Source: CAD feature listing. Evaluate the final solid. Frame: model axes, mm. A direction names the side the tool comes from. Round coordinates to 2 decimals unless told otherwise and drop trailing zeros. Order: outer loops, then holes, each group sorted by start corner. A loop starts at its lowest first (then second) coordinate and runs counter-clockwise, first axis right, second up. Notation, with made-up numbers: M 71,-4 L 109,-4 A11 ccw 109,11 Z; hole C 1,-16.5 d4. An arc over 180 degrees is marked long. Answer as CSV lines item,"result". Start each with the question number.
Item 1: First-contact query: P1, Ø3.5, axis at x = 0, y = 0, coming from the +Z side; P2, Ø2.5, axis at x = 0, y = 0, coming from the -Z side; P3, Ø2, axis at y = -2, z = 32, coming from the -X side; P4, Ø2, axis at x = 2, z = 22.5, coming from the -Y side. Flat tips, straight axial feed; report the tip coordinate or a pass-through.
Item 2: Set-up query: faces 1 (the face through (0, 0, 29)), 2 (the face through (0, 0, 6)), 3 (the face through (1.2, -1.2, 0)). Return all of +Z, -Z, +X, -X, +Y, -Y with unobstructed straight access to the full face (end or side cutting, diameter ignored); none if empty.
Item 3: Section query A-A on y = 0. Return the cut outline in (x, z), plus the area to 3 significant figures.
Item 4: Line query: line 1 (Y direction, x = 0, z = 37.75); line 2 (Z direction, x = 0.25, y = -0.5); line 3 (X direction, y = -0.75, z = 41.5). Output: solid intervals per line, ascending. Write a range as [from, to].
Item 5: Pull-direction query (X, two-part tool) for faces 4 (the face through (1.2, -1.2, 45)), 5 (the face through (-1.5, -0.07, 2.96)), 6 (the face through (-1.5, -0.07, 36.89)), 7 (the face through (-3, 0, 22)); classes: +X half, -X half, draft (parallel to the pull), parting line (faces both ways), or undercut.
Item 6: Section query D-D on z = 15. Return the cut outline in (x, y), plus the area to 3 significant figures.
Item 7: Section query C-C on z = 36. Return the cut outline in (x, y), plus the area to 3 significant figures.
Autodesk Inventor part; units mm, degrees
ref_plane "YZ Plane" through (0, 0, 0) normal (1, 0, 0) x (0, 1, 0)
ref_plane "XZ Plane" through (0, 0, 0) normal (0, 1, 0) x (-1, 0, 0)
ref_plane "XY Plane" through (0, 0, 0) normal (0, 0, 1) x (1, 0, 0)
sketch "スケッチ1" plane through (0, 0, 0) normal (0, 0, 1) x (1, 0, 0)
  circle A0 centre (0, 0) radius 3
  circle A1 centre (0, 0) radius 1.5
  dimension "d0" = 6
  dimension "d1" = 3
extrude "押し出し1" add sketch "スケッチ1" along normal blind 45
fillet "フィレット1" radius 0.3 2 edges at (-3, 0, 45) (-3, 0, 0)
thread "ねじ1"
extrude "押し出し2" add sketch "スケッチ1" along normal blind 29 contours A1
extrude "押し出し3" cut sketch "スケッチ1" along normal blind 6 contours A1
thread "ねじ2"
properties part number "スペーサーM3L45アルミ" material "アルミニウム 2014-T4"
Results:
1,P1,"z = 45"
1,P2,"z = 6"
1,P3,"x = -2.83"
1,P4,"y = -2.83"
2,face 1,"+Z"
2,face 2,"-Z"
2,face 3,"-Z, +X, -X, +Y, -Y"
3,outline,"M -3,0.3 A0.3 ccw -2.7,0 L -1.5,0 L -1.5,6 L 1.5,6 L 1.5,0 L 2.7,0 A0.3 ccw 3,0.3 L 3,44.7 A0.3 ccw 2.7,45 L 1.5,45 L 1.5,29 L -1.5,29 L -1.5,45 L -2.7,45 A0.3 ccw -3,44.7 Z"
3,area,"204 mm^2"
4,line 1,"[-3, -1.5], [1.5, 3]"
4,line 2,"[6, 29]"
4,line 3,"[-2.9, -1.3], [1.3, 2.9]"
5,face 4,"draft"
5,face 5,"undercut"
5,face 6,"undercut"
5,face 7,"parting line"
6,outline,"C 0,0 d6"
6,area,"28.3 mm^2"
7,outline,"C 0,0 d6; hole C 0,0 d3"
7,area,"21.2 mm^2"
